from build123d import *

# Parameters (mm, degrees)
F1_DEPTH   = 96.52
F2_W       = 90.17
F2_H       = 90.17
F3_DEPTH   = 106.68
F4_W       = 90.17
F4_H       = 90.17
F5_DEPTH   = 194.945
F8_D       = 19.05
F8_ON_F6_D = 19.05


with BuildPart() as f1:
    # F0 (on Top) → F1 (new body)
    with BuildSketch(Plane.XY):
        Polygon((198.12, 0), (0, 0), (0, -198.12), (96.52, -198.12), (96.52, -96.52), (198.12, -96.52), align=None)
    extrude(amount=F1_DEPTH)

    # F2 (on face) → F3 (cut)
    with BuildSketch(Plane.XZ.offset(198.12)):
        with Locations((48.26, 48.26)):
            Rectangle(F2_W, F2_H)
    extrude(amount=-F3_DEPTH, mode=Mode.SUBTRACT)

    # F4 (on face) → F5 (cut, through all)
    with BuildSketch(Plane.YZ.offset(198.12)):
        with Locations((-48.26, 48.26)):
            Rectangle(F4_W, F4_H)
    extrude(amount=-F5_DEPTH, mode=Mode.SUBTRACT)

    # F8 (through all)
    with Locations(Plane(origin=(0, 0, 0), x_dir=(-1, 0, 0), z_dir=(0, 1, 0))):
        with Locations((-134.62, 48.26)):
            Hole(F8_D / 2)

    # F8 on F6 (through all)
    with Locations(Plane(origin=(0, 0, 0), x_dir=(0, -1, 0), z_dir=(-1, 0, 0))):
        with Locations((134.62, 48.26)):
            Hole(F8_ON_F6_D / 2)


solid = f1.part
Read the model definition and answer for the solid it produces. Units are mm, in the model's axes. A direction names the side the tool comes from. Coordinates: 2 decimals unless noted, no trailing zeros. Write each loop counter-clockwise with the first axis right and the second up, starting at its lowest first coordinate (ties: lowest second). Pieces come first, ordered by that corner, then holes. Notation, with made-up numbers: M -11.5,16.25 L 6.5,16.25 A30 cw 6.5,51.25 Z; hole C -38.75,63.5 d8. An arc over 180 degrees is marked long. Use a Markdown table: item, result.
Q1. Determine the mould class of faces 4 (the face through (76, -76, 0)), 5 (the face through (94.955, -125.535, 51.121)), 6 (the face through (146, -93.345, 48)), 7 (the face through (100, 0, 48)) for opening direction Y: released by +Y, released by -Y, zero draft, split by the parting line, or undercut.
Answer block:
| item | result |
|---|---|
| face 4 | zero draft |
| face 5 | undercut |
| face 6 | undercut |
| face 7 | released by +Y |
Q2. Which of the six approach directions +Z, -Z, +X, -X, +Y, -Y give full straight-line access (tool end or side, diameter ignored) to faces 1 (the face through (147, -96.52, 48)), 2 (the face through (3.175, -102, 49)), 3 (the face through (80, -80, 3.175))?
Answer block:
| item | result |
|---|---|
| face 1 | +Z, -Z, +X, -Y |
| face 2 | -Y |
| face 3 | none |
Q3. The part is cut by section D-D, the plane z = 48.26. Write down the section's boundary in (x, y) (3 decimals).
Answer block:
| item | result |
|---|---|
| outline | M 0,-198.12 L 3.175,-198.12 L 3.175,-144.145 L 0,-144.145 Z; M 0,-125.095 L 3.175,-125.095 L 3.175,-3.175 L 125.095,-3.175 L 125.095,0 L 0,0 Z; M 93.345,-198.12 L 96.52,-198.12 L 96.52,-144.145 L 93.345,-144.145 Z; M 93.345,-125.095 L 96.52,-125.095 L 96.52,-96.52 L 125.095,-96.52 L 125.095,-93.345 L 93.345,-93.345 Z; M 144.145,-96.52 L 198.12,-96.52 L 198.12,-93.345 L 144.145,-93.345 Z; M 144.145,-3.175 L 198.12,-3.175 L 198.12,0 L 144.145,0 Z |
Q4. The part is cut by section C-C, the plane z = 28.5. Write down the section's boundary in (x, y) (3 decimals).
Answer block:
| item | result |
|---|---|
| outline | M 0,-198.12 L 3.175,-198.12 L 3.175,-3.175 L 198.12,-3.175 L 198.12,0 L 0,0 Z; M 93.345,-198.12 L 96.52,-198.12 L 96.52,-96.52 L 198.12,-96.52 L 198.12,-93.345 L 93.345,-93.345 Z |
Q5. Straight lines are drawn through the part: L1, parallel to Y at x = 165.5, z = 60 (3 decimals); L2, parallel to X at y = -190, z = 52.5 (3 decimals). For each, find the intervals that lie inside material, in ascending order. Write a range as [from, to].
Answer block:
| item | result |
|---|---|
| L1 | y = [-96.52, -93.345], [-3.175, 0] |
| L2 | x = [0, 3.175], [93.345, 96.52] |
Q6. The part is cut by section B-B, the plane x = 134.62. Write down the section's boundary in (y, z) (3 decimals).
Answer block:
| item | result |
|---|---|
| outline | M -96.52,0 L 0,0 L 0,38.735 L -3.175,38.735 L -3.175,3.175 L -93.345,3.175 L -93.345,38.735 L -96.52,38.735 Z; M -96.52,57.785 L -93.345,57.785 L -93.345,93.345 L -3.175,93.345 L -3.175,57.785 L 0,57.785 L 0,96.52 L -96.52,96.52 Z |
Q7. Each of these flat-tipped pins is pushed along its axis until it touches: pin 1 Ø25 at (x, z) = (134.62, 48.26) entering from -Y; pin 2 Ø17 at (x, z) = (134.62, 48.26) entering from -Y; pin 3 Ø6 at (x, z) = (67.5, 54.5) entering from -Y (3 decimals); pin 4 Ø25 at (y, z) = (-134.62, 48.26) entering from +X. Where does it stop, or does it pass through?
Answer block:
| item | result |
|---|---|
| pin 1 | stops at y = -96.52 |
| pin 2 | passes through |
| pin 3 | stops at y = -3.175 |
| pin 4 | stops at x = 96.52 |
Q8. The part is cut by section A-A, the plane y = -134.62. Write down the section's boundary in (x, z) (3 decimals).
Answer block:
| item | result |
|---|---|
| outline | M 0,0 L 96.52,0 L 96.52,38.735 L 93.345,38.735 L 93.345,3.175 L 3.175,3.175 L 3.175,38.735 L 0,38.735 Z; M 0,57.785 L 3.175,57.785 L 3.175,93.345 L 93.345,93.345 L 93.345,57.785 L 96.52,57.785 L 96.52,96.52 L 0,96.52 Z |
